Verification items for the finished model (mm, model axes). A direction names the side the tool comes from. Coordinates: 2 decimals unless noted, no trailing zeros. Order: outer loops, then holes, each group sorted by start corner. A loop starts at its lowest first (then second) coordinate and runs counter-clockwise, first axis right, second up.
Q1. Depth check by flat-ended pin: P1, Ø3, axis at y = -3.5, z = 36, coming from the +X side; P2, Ø2.5, axis at y = 6, z = 39.5, coming from the +X side; P3, Ø12, axis at x = -10.5, z = 3, coming from the -Y side. Enter the tip coordinate at first touch or a pass-through.
Q2. Cross-section at A-A, the plane x = -15. Record the boundary of the cut face in (y, z).
Q3. Cross-section at D-D, the plane y = 0.75. Record the boundary of the cut face in (x, z).
Q4. Cross-section at B-B, the plane z = 35. Record the boundary of the cut face in (x, y), and give its area (3 significant figures).
Q5. Thickness scan on line 1 (X direction, y = 11.65, z = 35); line 2 (Z direction, x = 15, y = 13.65); line 3 (X direction, y = 6, z = 1). Record the ranges inside material, lowest first.
Q6. Cross-section at C-C, the plane z = 25. Record the boundary of the cut face in (x, y).
Q7. Set-up check for faces 1 (the flat face through (-10.5, 7, 19)), 2 (the flat face through (12.5, 5, 20)), 3 (the cylindrical face through (0, -4, 39)), 4 (the flat face through (-12.5, 5, 20)): record each of +Z, -Z, +X, -X, +Y, -Y from which the full face is reachable in a straight line by a thin tool's end or side.
from build123d import *

# Parameters (mm, degrees)
SALIENTE_EXTRUIR1_DEPTH = 38
SALIENTE_EXTRUIR2_DEPTH = 3
SALIENTE_EXTRUIR3_DEPTH = 2
CROQUIS4_R              = 1.5
SALIENTE_EXTRUIR4_DEPTH = 4


with BuildPart() as part:
    # Croquis1 → Saliente-Extruir1 (new body)
    with BuildSketch(Plane.XY):
        with BuildLine():
            Line((-10.5, 0), (-10.5, 10.5))
            Line((-10.5, 10.5), (-12.5, 10.5))
            Line((-12.5, 10.5), (-12.5, 0))
            ThreePointArc((-12.5, 0), (0, -12.5), (12.5, 0))
            Line((12.5, 0), (12.5, 10.5))
            Line((12.5, 10.5), (10.5, 10.5))
            Line((10.5, 10.5), (10.5, 0))
            ThreePointArc((10.5, 0), (0, -10.5), (-10.5, 0))
        make_face()
    extrude(amount=SALIENTE_EXTRUIR1_DEPTH)

    # Croquis2 → Saliente-Extruir2 (add)
    with BuildSketch(Plane.XY.offset(38)):
        with BuildLine():
            Line((-12.5, 10.5), (-4, 10.5))
            Line((-4, 10.5), (-4, 0))
            ThreePointArc((-4, 0), (0, -4), (4, 0))
            Line((4, 0), (4, 10.5))
            Line((4, 10.5), (12.5, 10.5))
            Line((12.5, 10.5), (12.5, 0))
            ThreePointArc((12.5, 0), (0, -12.5), (-12.5, 0))
            Line((-12.5, 0), (-12.5, 10.5))
        make_face()
    extrude(amount=SALIENTE_EXTRUIR2_DEPTH)

    # Croquis3 → Saliente-Extruir3 (add)
    with BuildSketch(Plane(origin=(0, 0, 0), x_dir=(-1, 0, 0), z_dir=(0, 0, -1))):
        with BuildLine():
            Line((-12.5, 10.5), (12.5, 10.5))
            Line((12.5, 10.5), (12.5, 0))
            ThreePointArc((12.5, 0), (0, -12.5), (-12.5, 0))
            Line((-12.5, 0), (-12.5, 10.5))
        make_face()
    extrude(amount=SALIENTE_EXTRUIR3_DEPTH)

    # Croquis4 → Saliente-Extruir4 (add)
    with BuildSketch(Plane(origin=(0, 10.5, 0), x_dir=(1, 0, 0), z_dir=(0, 1, 0))):
        Polygon((-17.5, 2), (17.5, 2), (17.5, -41), (4, -41), (4, -38), (10.5, -38), (10.5, 0), (-10.5, 0), (-10.5, -38), (-4, -38), (-4, -41), (-17.5, -41), align=None)
        with Locations((-15, -3)):
            Circle(CROQUIS4_R, mode=Mode.SUBTRACT)
        with Locations((15, -3)):
            Circle(CROQUIS4_R, mode=Mode.SUBTRACT)
        with Locations((15, -35)):
            Circle(CROQUIS4_R, mode=Mode.SUBTRACT)
        with Locations((-15, -35)):
            Circle(CROQUIS4_R, mode=Mode.SUBTRACT)
    extrude(amount=SALIENTE_EXTRUIR4_DEPTH)


solid = part.part
Check values:
1. P1: stops at x = 12.34
1. P2: stops at x = 12.5
1. P3: stops at y = -11.66
2. outline: (10.5, -2) - (14.5, -2) - (14.5, 1.5) - (10.5, 1.5) - close; (10.5, 4.5) - (14.5, 4.5) - (14.5, 33.5) - (10.5, 33.5) - close; (10.5, 36.5) - (14.5, 36.5) - (14.5, 41) - (10.5, 41) - close
3. outline: (-12.5, -2) - (12.5, -2) - (12.5, 41) - (4, 41) - (4, 38) - (10.5, 38) - (10.5, 0) - (-10.5, 0) - (-10.5, 38) - (-4, 38) - (-4, 41) - (-12.5, 41) - close
4. outline: (-17.5, 10.5) - (-16.5, 10.5) - (-16.5, 14.5) - (-17.5, 14.5) - close; (-13.5, 10.5) - (-12.5, 10.5) - (-12.5, 0) arc R12.5 ccw to (12.5, 0) - (12.5, 10.5) - (13.5, 10.5) - (13.5, 14.5) - (10.5, 14.5) - (10.5, 0) arc R10.5 cw to (-10.5, 0) - (-10.5, 14.5) - (-13.5, 14.5) - close; (16.5, 10.5) - (17.5, 10.5) - (17.5, 14.5) - (16.5, 14.5) - close
4. area: 146 mm2
5. line 1: x = -17.5 to -16.5, -13.5 to -10.5, 10.5 to 13.5, 16.5 to 17.5
5. line 2: z = -2 to 1.5, 4.5 to 33.5, 36.5 to 41
5. line 3: x = -12.5 to -10.5, 10.5 to 12.5
6. outline: (-17.5, 10.5) - (-12.5, 10.5) - (-12.5, 0) arc R12.5 ccw to (12.5, 0) - (12.5, 10.5) - (17.5, 10.5) - (17.5, 14.5) - (10.5, 14.5) - (10.5, 0) arc R10.5 cw to (-10.5, 0) - (-10.5, 14.5) - (-17.5, 14.5) - close
7. face 1: +Y
7. face 2: +Z, -Z, +X, -Y
7. face 3: +Z, +Y
7. face 4: +Z, -Z, -X, -Y
